Work out the finished part from the listing and answer in its coordinate system (mm). Face numbers are marked on the shaded views. A direction names the side the tool comes from. Coordinates: 2 decimals unless noted, no trailing zeros. Write each loop counter-clockwise with the first axis right and the second up, starting at its lowest first coordinate (ties: lowest second). Pieces come first, ordered by that corner, then holes. Notation, with made-up numbers: (27, 70.25) - (54, 70.25) arc R23 ccw to (54, 100.25) - close; hole circle Ø5 at (-19, 45). An arc over 180 degrees is marked (long way). Use one line per item in the form item = value. Start each with the question number.
Item 1: A cutting plane is placed at C-C (x = -6.5). Write down the section's boundary in (y, z).
Item 2: A cutting plane is placed at D-D (y = 14). Write down the section's boundary in (x, z).
Item 3: A cutting plane is placed at B-B (y = 52.5). Write down the section's boundary in (x, z).
Item 4: Given pin 1 (5 mm diameter, centred on y = 62, z = -1.5, fed in from +X); pin 2 (4 mm diameter, centred on x = -14, z = 15.5, fed in from +Y); pin 3 (1 mm diameter, centred on x = 19, y = 25.5, fed in from -Z), each flat-ended and moving along its own axis, determine where each tip first touches the part or whether it passes through.
Item 5: Determine the mould class of the marked faces 1, 2 and 3 for opening direction Y: released by +Y, released by -Y, zero draft, split by the parting line, or undercut.
Item 6: For the marked faces 4, 5, 6 and 7, determine the directions among +Z, -Z, +X, -X, +Y, -Y from which every point of the face is accessible in a straight line to the end or side of a thin tool.
Item 7: A cutting plane is placed at A-A (z = 14.5). Write down the section's boundary in (x, y).
Item 8: Consider probe 1 along X at (y, z) = (50, 18.5); probe 2 along Y at (x, z) = (2, 13); probe 3 along Y at (x, z) = (-2, -18.5). Determine where each line is inside the solid, lowest interval first.
Autodesk Inventor part; units mm, degrees
ref_plane "YZ Plane" through (0, 0, 0) normal (1, 0, 0) x (0, 1, 0)
ref_plane "XZ Plane" through (0, 0, 0) normal (0, 1, 0) x (-1, 0, 0)
ref_plane "XY Plane" through (0, 0, 0) normal (0, 0, 1) x (1, 0, 0)
sketch "Sketch1" plane through (0, 0, 0) normal (0, 0, 1) x (1, 0, 0)
  line L0 (-45, 0) -> (45, 0)
  circle A0 centre (0.1619, 49.6388) radius 8
  circle A1 centre (0.1619, 49.6388) radius 20
  line L1 (-7.7534, 57.876) -> (-7.7534, 68.0058)
  line L2 (-7.7534, 57.876) -> (-18.063, 57.876)
  line L3 (8.2464, 58) -> (18.3303, 58)
  line L4 (8.2464, 58) -> (8.2464, 67.932)
  line L5 (25, 58) -> (18.3303, 58)
  line L6 (-24.7326, 57.9068) -> (-18.063, 57.876)
  line L7 (45, 0) -> (-45, 0)
  line L8 (-41.85, 9) -> (-41.85, 45)
  line L9 (-41.85, 45) -> (-29.25, 45)
  line L10 (41.8966, 9) -> (41.8966, 45)
  line L11 (41.8966, 45) -> (29.4828, 45)
  line L12 (-38, 20) -> (38, 20)
  line L13 (-45, 0) -> (-24.7326, 57.9068)
  line L14 (25, 58) -> (45, 0)
  line L15 (-45, 0) -> (-38, 20)
  line L16 (38, 20) -> (45, 0)
  point P0 (0, 0)
extrude "Extrusion1" add sketch "Sketch1" along normal mid plane 44 contours A1 L2 L1 L4 L3
extrude "Extrusion2" add sketch "Sketch1" along normal mid plane 44 contours L3 L4 A1
extrude "Extrusion3" add sketch "Sketch1" along normal mid plane 44 contours A1 L1 L2
extrude "Extrusion4" cut sketch "Sketch1" along normal mid plane 24 contours A1 L1 L2
extrude "Extrusion5" cut sketch "Sketch1" along normal mid plane 24 contours L3 L4 A1
extrude "Extrusion6" add sketch "Sketch1" along normal mid plane 16 contours L14 L11 L10
extrude "Extrusion7" add sketch "Sketch1" along normal mid plane 16 contours L8 L9 L13
extrude "Extrusion8" add sketch "Sketch1" along normal mid plane 24 contours L16 L12 L13 L6 A1 L5 L14
extrude "Extrusion9" add sketch "Sketch1" along normal mid plane 60 contours L13 L12 L16 L0
properties part number "Q2 auto"
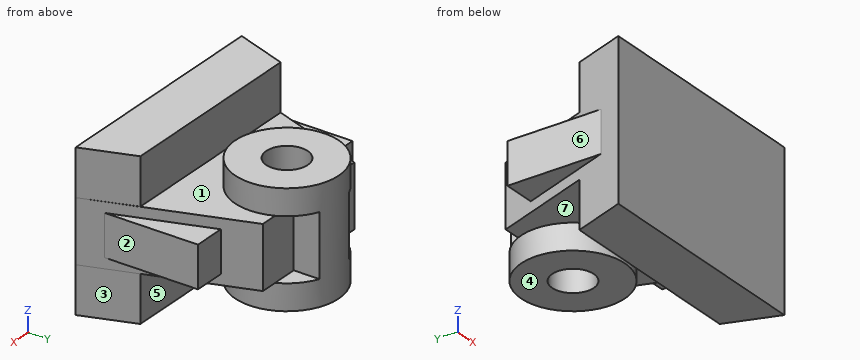
Answer:
q1.outline = (0, -30) - (20, -30) - (20, -12) - (30.78, -12) - (30.78, -22) - (45.21, -22) - (45.21, 22) - (30.78, 22) - (30.78, 12) - (20, 12) - (20, 30) - (0, 30) - close; (54.07, -22) - (68.5, -22) - (68.5, 22) - (54.07, 22) - close
q2.outline = (-41.85, -8) - (-40.1, -8) - (-40.1, -30) - (40.1, -30) - (40.1, -12) - (40.17, -12) - (40.17, -8) - (41.9, -8) - (41.9, 8) - (40.17, 8) - (40.17, 12) - (40.1, 12) - (40.1, 30) - (-40.1, 30) - (-40.1, 8) - (-41.85, 8) - close
q3.outline = (-26.62, -12) - (-19.63, -12) - (-19.63, -22) - (-7.31, -22) - (-7.31, 22) - (-19.63, 22) - (-19.63, 12) - (-26.62, 12) - close; (7.63, -22) - (19.96, -22) - (19.96, -12) - (26.9, -12) - (26.9, 12) - (19.96, 12) - (19.96, 22) - (7.63, 22) - close
q4.pin_1 = 8.25
q4.pin_2 = 65.52
q4.pin_3 = -12
q5.face_1 = undercut
q5.face_2 = zero draft
q5.face_3 = released by +Y
q6.face_4 = -Z, +X, -X, +Y
q6.face_5 = -Z, +X, -X
q6.face_6 = +Z, -Z, -X, +Y
q6.face_7 = -Z
q7.outline = (-45, 0) - (45, 0) - (38, 20) - (-38, 20) - close; circle Ø40 at (0.16, 49.64); hole circle Ø16 at (0.16, 49.64)
q8.probe_1 = -19.83 to -7.83, 8.15 to 20.16
q8.probe_2 = 0 to 20, 29.72 to 41.85, 57.42 to 69.55
q8.probe_3 = 0 to 20, 29.76 to 41.94, 57.34 to 69.52
